from build123d import *

# Parameters (mm, degrees)
BOSS_EXTRUDE1_DEPTH      = 50
CUT_EXTRUDE1_DEPTH       = 100
BOSS_EXTRUDE2_DEPTH      = 40
BOSS_EXTRUDE2_DEPTH_BACK = 80
SKETCH5_R                = 6.133635391
SKETCH5_W                = 29.300165504
SKETCH5_H                = 7.581524949
CUT_EXTRUDE2_DEPTH       = 10
FILLET1_R                = 40
FILLET2_R                = 40
SKETCH6_R                = 9.612627596
SKETCH6_R_2              = 10.978592339
CUT_EXTRUDE3_DEPTH       = 10
SKETCH7_R                = 10.62877533
CUT_EXTRUDE4_DEPTH       = 20


with BuildPart() as part:
    # Sketch1 → Boss-Extrude1 (new body)
    with BuildSketch(Plane.XY):
        Polygon((34.876820554, 10.095921739), (-11.47263834, 66.541302373), (-50.93851423, 10.095921739), align=None)
    extrude(amount=-BOSS_EXTRUDE1_DEPTH)

    # Sketch2 → Cut-Extrude1 (cut)
    with BuildSketch(Plane(origin=(-38.95420386, 27.236272618, 0), x_dir=(0, 0, 1), z_dir=(-0.819544824, 0.57301508, 0))):
        Polygon((-37.846995644, 47.959585147), (-37.846995644, 28.259004522), (-23.196912892, 28.259004522), (-8.54683014, 28.259004522), (0, 28.259004522), (0, 47.959585147), align=None)
        Polygon((-8.54683014, 15.307343506), (-8.54683014, -20.914476405), (0, -20.914476405), (0, 28.259004522), (-8.54683014, 28.259004522), align=None)
        with BuildLine():
            ThreePointArc((-23.196912892, 28.259004522), (-13.419765459, 24.556838072), (-8.54683014, 15.307343506))
            Line((-8.54683014, 15.307343506), (-8.54683014, 28.259004522))
            Line((-8.54683014, 28.259004522), (-23.196912892, 28.259004522))
        make_face()
        with BuildLine():
            Line((-37.846995644, 28.259004522), (-37.846995644, 15.307343506))
            ThreePointArc((-37.846995644, 15.307343506), (-32.974060325, 24.556838072), (-23.196912892, 28.259004522))
            Line((-23.196912892, 28.259004522), (-37.846995644, 28.259004522))
        make_face()
        Polygon((-50, -20.914476405), (-37.846995644, -20.914476405), (-37.846995644, 15.307343506), (-37.846995644, 28.259004522), (-37.846995644, 47.959585147), (-50, 47.959585147), align=None)
    extrude(amount=-CUT_EXTRUDE1_DEPTH, mode=Mode.SUBTRACT)

    # Sketch3 → Boss-Extrude2 (add, two sides)
    with BuildSketch(Plane.XY) as boss_extrude2_sk:
        Polygon((149.486050835, 10.095921739), (-50.93851423, 10.095921739), (-50.93851423, -94.77972655), (-40.577313053, -94.77972655), (-40.577313053, 0), (149.486050835, 0), align=None)
    extrude(amount=BOSS_EXTRUDE2_DEPTH)
    extrude(boss_extrude2_sk.sketch, amount=-BOSS_EXTRUDE2_DEPTH_BACK)

    # Sketch5 → Cut-Extrude2 (cut)
    with BuildSketch(Plane(origin=(-38.95420386, 27.236272618, 0), x_dir=(0, 0, 1), z_dir=(-0.819544824, 0.57301508, 0))):
        with Locations((-23.196912892, 13.497560131)):
            Circle(SKETCH5_R)
        with Locations((-23.196912892, -6.594328923)):
            Rectangle(SKETCH5_W, SKETCH5_H)
    extrude(amount=-CUT_EXTRUDE2_DEPTH, mode=Mode.SUBTRACT)

    # Fillet1
    fillet1_edges = [part.edges().sort_by_distance(p)[0] for p in [
        (-45.757913642, -94.77972655, -80),
        (-45.757913642, -94.77972655, 40),
    ]]
    fillet(fillet1_edges, radius=FILLET1_R)

    # Fillet2
    fillet2_edges = [part.edges().sort_by_distance(p)[0] for p in [
        (149.486050835, 5.04796087, -80),
        (149.486050835, 5.04796087, 40),
    ]]
    fillet(fillet2_edges, radius=FILLET2_R)

    # Sketch6 → Cut-Extrude3 (cut)
    with BuildSketch(Plane(origin=(0, 10.095921739, 0), x_dir=(1, 0, 0), z_dir=(0, 1, 0))):
        with Locations((109.486050835, 59.137142256)):
            Circle(SKETCH6_R)
        with Locations((109.486050835, -18.771374572)):
            Circle(SKETCH6_R_2)
    extrude(amount=-CUT_EXTRUDE3_DEPTH, mode=Mode.SUBTRACT)

    # Sketch7 → Cut-Extrude4 (cut)
    with BuildSketch(Plane.ZY.offset(50.93851423)):
        with Locations((-63.54369248, -57.164065998)):
            Circle(SKETCH7_R)
        with Locations((24.915147361, -57.164065998)):
            Circle(SKETCH7_R)
    extrude(amount=-CUT_EXTRUDE4_DEPTH, mode=Mode.SUBTRACT)


solid = part.part
Geometry check sheet. Reference: the model listing, model coordinates, mm. A direction names the side the tool comes from. Round coordinates to 2 decimals unless told otherwise and drop trailing zeros. Loops run counter-clockwise (first coordinate to the right, second up) from the corner with the lowest first, then second, coordinate; pieces in that order, holes last. Notation, with made-up numbers: (54, 84) -> (63, 84) arc R25 cw to (63, 103) -> close; hole circle Ø2 at (77.5, 18). An arc over 180 degrees is marked (long way). Answer as a JSON object with one key per item and string values. Group by question number.
Item 1: Cross-section at A-A, the plane z = 24. Record the cut outline in (x, y).
Item 2: Cross-section at D-D, the plane y = -28. Record the cut outline in (x, z).
Item 3: Cross-section at B-B, the plane z = -33.5. Record the cut outline in (x, y).
Item 4: Depth check by flat-ended pin: pin 1 Ø2 at (y, z) = (-13, -38) entering from +X; pin 2 Ø12 at (x, z) = (-11, -60) entering from -Y; pin 3 Ø17.5 at (x, z) = (109.5, 19.5) entering from +Y. Enter the tip coordinate at first touch or a pass-through.
Item 5: Cross-section at C-C, the plane x = 91.5. Record the cut outline in (y, z).
Item 6: Release check for a two-part mould opening along X. For faces 1 (the face through (-27.025, 35.694, -29.325)), 2 (the face through (-40.865, 15.9, -23.402)), 3 (the face through (-45.685, -82.751, 28.594)), 4 (the face through (137.46, 5.12, -68.59)) record: pulls with the +X half, pulls with the -X half, needs draft (parallel to the pull), parting line crosses it, or undercut.
Item 7: Set-up check for faces 5 (the face through (98.52, 5.17, 18.29)), 6 (the face through (-20, 20, -37.847)), 7 (the face through (-22, 17, -8.547)): record each of +Z, -Z, +X, -X, +Y, -Y from which the full face is reachable in a straight line by a thin tool's end or side.
Item 8: Thickness scan on line 1 along X through (y, z) = (-20, 11); line 2 along Y through (x, z) = (23, -38.5); line 3 along Z through (x, y) = (-13.5, 28). Record the ranges inside material, lowest first.
Determined:
{
 "1": {"outline": "(-50.94, -86.78) -> (-40.58, -86.78) -> (-40.58, -67.75) -> (-50.94, -67.75) -> close; (-50.94, -46.57) -> (-40.58, -46.57) -> (-40.58, 0) -> (141.49, 0) -> (141.49, 10.1) -> (119.14, 10.1) -> (119.14, 0.1) -> (99.83, 0.1) -> (99.83, 10.1) -> (-50.94, 10.1) -> close"},
 "2": {"outline": "(-50.94, -80) -> (-40.58, -80) -> (-40.58, 40) -> (-50.94, 40) -> close"},
 "3": {"outline": "(-50.94, -94.78) -> (-40.58, -94.78) -> (-40.58, 0) -> (149.49, 0) -> (149.49, 10.1) -> (27.56, 10.1) -> (-25.16, 46.96) -> (-40.56, 24.94) -> (-32.37, 19.21) -> (-36.71, 13) -> (-44.91, 18.73) -> (-50.94, 10.1) -> close"},
 "4": {"pin 1": "stops at x = -40.58", "pin 2": "stops at y = 0", "pin 3": "stops at y = 0.1"},
 "5": {"outline": "(0, -80) -> (10.1, -80) -> (10.1, 40) -> (0, 40) -> close"},
 "6": {"face 1": "undercut", "face 2": "undercut", "face 3": "needs draft", "face 4": "pulls with the +X half"},
 "7": {"face 5": "+Y", "face 6": "-Z, +X, -X, +Y", "face 7": "+Z, +X, -X, +Y"},
 "8": {"line 1": "x = -50.94 to -40.58", "line 2": "y = 0 to 10.1", "line 3": "z = -37.85 to -8.55"}
}
